Geometry check sheet. Reference: the model listing, model coordinates, mm. A direction names the side the tool comes from. Give positions to 0.01 mm unless a question says otherwise; leave off trailing zeros. Write each loop counter-clockwise with the first axis right and the second up, starting at its lowest first coordinate (ties: lowest second). Pieces come first, ordered by that corner, then holes. Notation, with made-up numbers: (76.25, 73) - (114.25, 73) arc R20 ccw to (114.25, 99) - close; hole circle Ø8 at (20, 55). An arc over 180 degrees is marked (long way). Write item = value, one per line. Start each with the question number.
(1) Section check A-A, the plane y = 10. Enter the section's corners in (x, z), plus the area to 3 significant figures.
(2) Section check C-C, the plane z = 6. Give the number of separate pieces and of enclosed holes in the cut face, plus the area to 3 significant figures.
(3) Access from +Z, -Z, +X, -X, +Y, -Y to the whole of each face (thin tool, end or side, straight path). Record for faces 4 (the flat face through (9, -5, 9)), 5 (the flat face through (8.46, -8.37, 5.96)), 6 (the flat face through (-10.637, -6.109, 5.958)), 7 (the flat face through (0, 12.267, 3.2)), 8 (the cylindrical face through (15.336, 4.838, 1.479)).
(4) Section check D-D, the plane y = 0. Enter the section's corners in (x, z).
(5) Thickness scan on L1, parallel to X at y = 3, z = 0.75; L2, parallel to Z at x = 0, y = -9.65; L3, parallel to Z at x = -5, y = -12. Record the ranges inside material, lowest first.
(6) Draft check along Z on faces 1 (the cylindrical face through (10.862, 10.86, 1.479)), 2 (the flat face through (8, -4, 0)), 3 (the flat face through (0, 10, 9)). Enter one of: pulls with the +Z half, pulls with the -Z half, needs draft (parallel to the pull), parting line crosses it, or undercut.
(7) Depth check by flat-ended pin: pin 1 Ø2 at (y, z) = (-9.5, 7.5) entering from -X; pin 2 Ø2.5 at (x, z) = (0, 6) entering from +Y; pin 3 Ø4 at (x, z) = (0, 6) entering from +Y; pin 4 Ø0.5 at (x, z) = (1, 8.5) entering from -Y. Enter the tip coordinate at first touch or a pass-through.
(8) Section check B-B, the plane x = 0. Enter the section's corners in (y, z), plus the area to 3 significant figures.
```python
from build123d import *

# Parameters (mm, degrees)
F0_R          = 17.5
F0_R_2        = 11.5
F1_DEPTH      = 3
F3_DEPTH      = 3.001
F5_DEPTH      = 6
F5_DEPTH_BACK = 3
F6_R          = 1.5
F7_DEPTH      = 29.767666761


# Not quite as in the source:
# - a fillet or chamfer that OpenCascade refuses, or shapes differently, is made with other operations: its cross-section is extruded or revolved along the edge and cut away or added


with BuildPart() as f1:
    # F0 (on Top) → F1 (new body)
    with BuildSketch(Plane.XY):
        Circle(F0_R)
        Circle(F0_R_2, mode=Mode.SUBTRACT)
    extrude(amount=F1_DEPTH)

    # F2 (on Top) → F3 (cut, through all)
    with BuildSketch(Plane.XY):
        with BuildLine():
            ThreePointArc((10.3428791664, 8.0132342217), (10.722508829, 7.4074823165), (11.2842680034, 7.8496142891))
            ThreePointArc((11.2842680034, 7.8496142891), (10.8476709377, 10.9006538274), (9.2192751651, 13.5174813857))
            ThreePointArc((9.2192751651, 13.5174813857), (8.6315737781, 13.5584848298), (8.5342502168, 12.9774492654))
            ThreePointArc((8.5342502168, 12.9774492654), (9.9604845752, 10.6854945477), (10.3428791664, 8.0132342217))
        make_face()
        with BuildLine():
            ThreePointArc((2.7722974401, 12.7867681236), (3.4524804527, 12.5667564861), (3.5986159928, 13.2665410638))
            ThreePointArc((3.5986159928, 13.2665410638), (1.3029928249, 15.3231337636), (-1.6264950391, 16.2810273468))
            ThreePointArc((-1.6264950391, 16.2810273468), (-2.1030569267, 15.9346706376), (-1.8041286384, 15.427013193))
            ThreePointArc((-1.8041286384, 15.427013193), (0.761670361, 14.5880397916), (2.7722974401, 12.7867681236))
        make_face()
        with BuildLine():
            ThreePointArc((-6.0954730691, 11.5772311114), (-5.4330018975, 11.8459056319), (-5.770868435, 12.4759058335))
            ThreePointArc((-5.770868435, 12.4759058335), (-8.8513701119, 12.5757491141), (-11.711210138, 11.426499669))
            ThreePointArc((-11.711210138, 11.426499669), (-11.8536439226, 10.85484696), (-11.298335653, 10.6581061954))
            ThreePointArc((-11.298335653, 10.6581061954), (-8.7935378801, 11.6646790891), (-6.0954730691, 11.5772311114))
        make_face()
        with BuildLine():
            ThreePointArc((-12.1111039857, 4.9505789955), (-11.7763222787, 5.5822238799), (-12.440099386, 5.8476556095))
            ThreePointArc((-12.440099386, 5.8476556095), (-14.8640786012, 3.9440316902), (-16.3161198577, 1.2253858046))
            ThreePointArc((-16.3161198577, 1.2253858046), (-16.0577791885, 0.6959197515), (-15.5059258486, 0.9021528573))
            ThreePointArc((-15.5059258486, 0.9021528573), (-14.2341520178, 3.2832854023), (-12.1111039857, 4.9505789955))
        make_face()
        with BuildLine():
            ThreePointArc((-12.4598147474, -3.9925040519), (-12.6093705865, -3.293442465), (-13.288469578, -3.5167776637))
            ThreePointArc((-13.288469578, -3.5167776637), (-13.9217195173, -6.5331419945), (-13.2865357625, -9.5490996964))
            ThreePointArc((-13.2865357625, -9.5490996964), (-12.7483011098, -9.7886360429), (-12.4581210104, -9.275927829))
            ThreePointArc((-12.4581210104, -9.275927829), (-13.0144482314, -6.6343940139), (-12.4598147474, -3.9925040519))
        make_face()
        with BuildLine():
            ThreePointArc((-6.9784397134, -11.0674500817), (-7.5423542593, -10.6280704779), (-7.9190171696, -11.2356715834))
            ThreePointArc((-7.9190171696, -11.2356715834), (-6.4652331485, -13.9533859322), (-4.0400339207, -15.855455323))
            ThreePointArc((-4.0400339207, -15.855455323), (-3.4737512602, -15.6929802443), (-3.5810228949, -15.1136987937))
            ThreePointArc((-3.5810228949, -15.1136987937), (-5.705139478, -13.4477667379), (-6.9784397134, -11.0674500817))
        make_face()
        with BuildLine():
            ThreePointArc((1.7682248193, -12.9638132172), (1.0538134497, -12.9897061964), (1.1558313826, -13.6972698986))
            ThreePointArc((1.1558313826, -13.6972698986), (4.0164076635, -14.8446855176), (7.0968446926, -14.7428671903))
            ThreePointArc((7.0968446926, -14.7428671903), (7.4262054104, -14.2544045814), (6.9716756317, -13.8796021227))
            ThreePointArc((6.9716756317, -13.8796021227), (4.2736674427, -13.9687799499), (1.7682248193, -12.9638132172))
        make_face()
        with BuildLine():
            ThreePointArc((9.6875173073, -8.7942640717), (9.1568901338, -9.2733140211), (9.6898535852, -9.7497634001))
            ThreePointArc((9.6898535852, -9.7497634001), (12.6187266924, -8.7899917691), (14.9130308016, -6.7319276504))
            ThreePointArc((14.9130308016, -6.7319276504), (14.8513580365, -6.1460345947), (14.2622496488, -6.151085364))
            ThreePointArc((14.2622496488, -6.151085364), (12.2527778705, -7.9536457777), (9.6875173073, -8.7942640717))
        make_face()
        with BuildLine():
            ThreePointArc((13.0739127825, -0.5097810297), (12.9753561567, -1.2178351539), (13.6898856045, -1.2402342502))
            ThreePointArc((13.6898856045, -1.2402342502), (15.3166032603, 1.3776368181), (15.7512440587, 4.4289556541))
            ThreePointArc((15.7512440587, 4.4289556541), (15.3273951828, 4.8381332844), (14.8793585479, 4.4555925983))
            ThreePointArc((14.8793585479, 4.4555925983), (14.4986773582, 1.7830876488), (13.0739127825, -0.5097810297))
        make_face()
    extrude(amount=F3_DEPTH, mode=Mode.SUBTRACT)

    # F4 (on face) → F5 (join, two sides)
    with BuildSketch(Plane.XY.offset(3)) as f5_sk:
        with BuildLine():
            ThreePointArc((-4, 10.7819293264), (0, 8), (4, 10.7819293264))
            ThreePointArc((4, 10.7819293264), (0, 11.5), (-4, 10.7819293264))
        make_face()
        with BuildLine():
            ThreePointArc((7.3374246985, 8.8550662783), (6.9282032303, 4), (11.3374246985, 1.9268630481))
            ThreePointArc((11.3374246985, 1.9268630481), (9.9592921435, 5.75), (7.3374246985, 8.8550662783))
        make_face()
        with BuildLine():
            ThreePointArc((7.3374246985, -8.8550662783), (9.9592921435, -5.75), (11.3374246985, -1.9268630481))
            ThreePointArc((11.3374246985, -1.9268630481), (6.9282032303, -4), (7.3374246985, -8.8550662783))
        make_face()
        with BuildLine():
            ThreePointArc((-4, -10.7819293264), (0, -11.5), (4, -10.7819293264))
            ThreePointArc((4, -10.7819293264), (0, -8), (-4, -10.7819293264))
        make_face()
        with BuildLine():
            ThreePointArc((-11.3374246985, -1.9268630481), (-9.9592921435, -5.75), (-7.3374246985, -8.8550662783))
            ThreePointArc((-7.3374246985, -8.8550662783), (-6.9282032303, -4), (-11.3374246985, -1.9268630481))
        make_face()
        with BuildLine():
            ThreePointArc((-11.3374246985, 1.9268630481), (-6.9282032303, 4), (-7.3374246985, 8.8550662783))
            ThreePointArc((-7.3374246985, 8.8550662783), (-9.9592921435, 5.75), (-11.3374246985, 1.9268630481))
        make_face()
        with BuildLine():
            ThreePointArc((-4, 10.7819293264), (0, 11.5), (4, 10.7819293264))
            Line((4, 10.7819293264), (2, 12.266666761))
            Line((2, 12.266666761), (0, 12.266666761))
            Line((0, 12.266666761), (-2, 12.266666761))
            Line((-2, 12.266666761), (-4, 10.7819293264))
        make_face()
        with BuildLine():
            ThreePointArc((7.3374246985, 8.8550662783), (9.9592921435, 5.75), (11.3374246985, 1.9268630481))
            Line((11.3374246985, 1.9268630481), (11.6232450348, 4.4012825729))
            Line((11.6232450348, 4.4012825729), (10.6232450348, 6.1333333805))
            Line((10.6232450348, 6.1333333805), (9.6232450348, 7.8653841881))
            Line((9.6232450348, 7.8653841881), (7.3374246985, 8.8550662783))
        make_face()
        with BuildLine():
            Line((11.6232450348, -4.4012825729), (11.3374246985, -1.9268630481))
            ThreePointArc((11.3374246985, -1.9268630481), (9.9592921435, -5.75), (7.3374246985, -8.8550662783))
            Line((7.3374246985, -8.8550662783), (9.6232450348, -7.8653841881))
            Line((9.6232450348, -7.8653841881), (10.6232450348, -6.1333333805))
            Line((10.6232450348, -6.1333333805), (11.6232450348, -4.4012825729))
        make_face()
        with BuildLine():
            Line((2, -12.266666761), (4, -10.7819293264))
            ThreePointArc((4, -10.7819293264), (0, -11.5), (-4, -10.7819293264))
            Line((-4, -10.7819293264), (-2, -12.266666761))
            Line((-2, -12.266666761), (0, -12.266666761))
            Line((0, -12.266666761), (2, -12.266666761))
        make_face()
        with BuildLine():
            Line((-9.6232450348, -7.8653841881), (-7.3374246985, -8.8550662783))
            ThreePointArc((-7.3374246985, -8.8550662783), (-9.9592921435, -5.75), (-11.3374246985, -1.9268630481))
            Line((-11.3374246985, -1.9268630481), (-11.6232450348, -4.4012825729))
            Line((-11.6232450348, -4.4012825729), (-10.6232450348, -6.1333333805))
            Line((-10.6232450348, -6.1333333805), (-9.6232450348, -7.8653841881))
        make_face()
        with BuildLine():
            ThreePointArc((-11.3374246985, 1.9268630481), (-9.9592921435, 5.75), (-7.3374246985, 8.8550662783))
            Line((-7.3374246985, 8.8550662783), (-9.6232450348, 7.8653841881))
            Line((-9.6232450348, 7.8653841881), (-10.6232450348, 6.1333333805))
            Line((-10.6232450348, 6.1333333805), (-11.6232450348, 4.4012825729))
            Line((-11.6232450348, 4.4012825729), (-11.3374246985, 1.9268630481))
        make_face()
    extrude(amount=F5_DEPTH)
    extrude(f5_sk.sketch, amount=-F5_DEPTH_BACK)

    # F6 (on face) → F7 (cut, through all)
    with BuildSketch(Plane.XZ.offset(12.266666761)):
        with Locations((0, 6)):
            Circle(F6_R)
    extrude(amount=-F7_DEPTH, mode=Mode.SUBTRACT)

    # F8: chamfer of 1 on 2 edges, made by hand

    # F8_s1 → F8_t2 (revolve, cut)
    with BuildSketch(Plane.XY.offset(6)):
        Polygon((2.5, -12.266666761), (1.5, -11.266666761), (1.5, -12.266666761), align=None)
    revolve(axis=Axis((0, -12.266666761, 6), (0, -1, 0)), mode=Mode.SUBTRACT)

    # F8_s3 → F8_t4 (revolve, cut)
    with BuildSketch(Plane.XY.offset(6)):
        Polygon((2.5, 12.266666761), (1.5, 11.266666761), (1.5, 12.266666761), align=None)
    revolve(axis=Axis((0, 12.266666761, 6), (0, -1, 0)), mode=Mode.SUBTRACT)


solid = f1.part
```
Model answer:
q1.outline = (-14.36, 0) - (-5.68, 0) - (-5.68, 3) - (-14.36, 3) - close; (-3.61, 0) - (3.61, 0) - (3.61, 9) - (-3.61, 9) - close; (5.68, 0) - (10.17, 0) - (10.17, 3) - (5.68, 3) - close; (11.11, 0) - (14.36, 0) - (14.36, 3) - (11.11, 3) - close; hole circle Ø3 at (0, 6)
q1.area = 107 mm²
q2.separate_pieces = 8
q2.enclosed_holes = 0
q2.area = 124 mm²
q3.face_4 = +Z, +X, -X, +Y, -Y
q3.face_5 = +Z, +X, -Y
q3.face_6 = +Z, -X, -Y
q3.face_7 = +Z, +X, -X, +Y
q3.face_8 = +Z, -Z
q4.outline = (-17.5, 0) - (-11.5, 0) - (-11.5, 3) - (-17.5, 3) - close; (11.5, 0) - (13.51, 0) - (13.51, 3) - (11.5, 3) - close; (14.65, 0) - (17.5, 0) - (17.5, 3) - (14.65, 3) - close
q5.L1 = -17.24 to -15.54, -14.46 to -7.73, 7.73 to 14.81, 15.71 to 17.24
q5.L2 = 0 to 4.5, 7.5 to 9
q5.L3 = 0 to 3
q6.face_1 = needs draft
q6.face_2 = pulls with the -Z half
q6.face_3 = pulls with the +Z half
q7.pin_1 = -8.16
q7.pin_2 = through
q7.pin_3 = 11.77
q7.pin_4 = -12.27
q8.outline = (-17.5, 0) - (-8, 0) - (-8, 4.5) - (-11.27, 4.5) - (-12.27, 3.5) - (-12.27, 3) - (-17.5, 3) - close; (-12.27, 8.5) - (-11.27, 7.5) - (-8, 7.5) - (-8, 9) - (-12.27, 9) - close; (8, 0) - (14.96, 0) - (14.96, 3) - (12.27, 3) - (12.27, 3.5) - (11.27, 4.5) - (8, 4.5) - close; (8, 7.5) - (11.27, 7.5) - (12.27, 8.5) - (12.27, 9) - (8, 9) - close; (15.92, 0) - (17.5, 0) - (17.5, 3) - (15.92, 3) - close
q8.area = 77.7 mm²
